Check sheet for the modelled part. Datum: model origin and axes. Units: mm. Face numbers are marked on the shaded views. Coordinates: 2 decimals unless noted, no trailing zeros. Loops run counter-clockwise (first coordinate to the right, second up) from the corner with the lowest first, then second, coordinate; pieces in that order, holes last. Notation, with made-up numbers: M -38,44 L -14,44 A30 ccw -14,75 Z; hole C 51.25,2.5 d2. An arc over 180 degrees is marked long. Use CSV: the item, a comma, the result in double quotes. Start each with the question number.
(1) Section check B-B on z = -15. Record the cut outline in (x, y), and give its area (3 significant figures).
(2) Section check A-A on x = 0. Record the cut outline in (y, z).
(3) Section check C-C on z = 0. Record the cut outline in (x, y).
(4) Go/stop test with flat-tipped pins: pin 1 Ø2.5 at (x, z) = (0, -15) entering from +Y (1 decimal); pin 2 Ø6.5 at (x, z) = (0, 15) entering from +Y; pin 3 Ø1 at (x, y) = (-3, 26) entering from +Z; pin 4 Ø10 at (y, z) = (21, 8) entering from -X. Record where each tip stops, or that it passes through.
(5) Section check D-D on y = -1. Record the cut outline in (x, z).
(6) Draft check along Z on the marked faces 1, 2 and 3. Enter one of: pulls with the +Z half, pulls with the -Z half, needs draft (parallel to the pull), parting line crosses it, or undercut.
(7) Scan lines: line 1 (Z direction, x = 0, y = -1.5); line 2 (X direction, y = 26, z = 0); line 3 (X direction, y = 0, z = 15). Record each from-to range of solid material in increasing order.
from build123d import *

# Parameters (mm, degrees)
SKETCH1_W           = 29
SKETCH1_H           = 7
BOSS_EXTRUDE1_DEPTH = 20
SKETCH2_R           = 2
CUT_EXTRUDE1_DEPTH  = 8
SKETCH3_R           = 7.75
SKETCH3_R_2         = 5.25
EXTRUDE_THIN1_DEPTH = 30


with BuildPart() as part:
    # Sketch1 → Boss-Extrude1 (new body, symmetric)
    with BuildSketch(Plane.XY):
        Rectangle(SKETCH1_W, SKETCH1_H)
    extrude(amount=BOSS_EXTRUDE1_DEPTH, both=True)

    # Sketch2 → Cut-Extrude1 (cut, through all)
    with BuildSketch(Plane(origin=(0, 3.5, 0), x_dir=(1, 0, 0), z_dir=(0, 1, 0))):
        with Locations((0, 15)):
            Circle(SKETCH2_R)
        with Locations((0, -15)):
            Circle(SKETCH2_R)
    extrude(amount=-CUT_EXTRUDE1_DEPTH, mode=Mode.SUBTRACT)

    # Sketch3 → Extrude-Thin1 (add)
    with BuildSketch(Plane(origin=(0, 3.5, 0), x_dir=(1, 0, 0), z_dir=(0, 1, 0))):
        Circle(SKETCH3_R)
        Circle(SKETCH3_R_2, mode=Mode.SUBTRACT)
    extrude(amount=EXTRUDE_THIN1_DEPTH)


solid = part.part
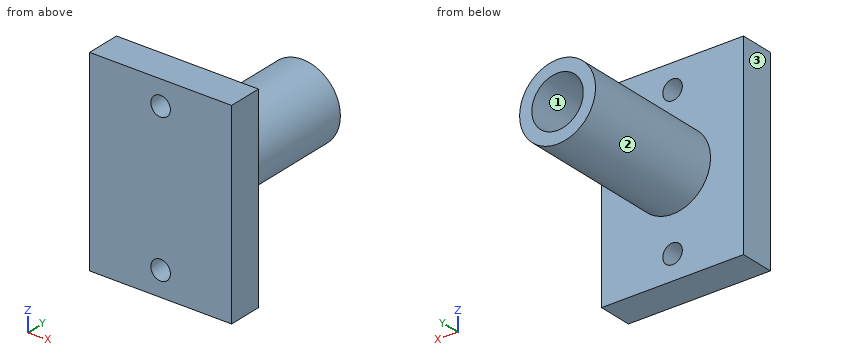
Outcome:
1,outline,"M -14.5,-3.5 L -2,-3.5 L -2,3.5 L -14.5,3.5 Z; M 2,-3.5 L 14.5,-3.5 L 14.5,3.5 L 2,3.5 Z"
1,area,"175 mm²"
2,outline,"M -3.5,-20 L 3.5,-20 L 3.5,-17 L -3.5,-17 Z; M -3.5,-13 L 3.5,-13 L 3.5,-7.75 L 33.5,-7.75 L 33.5,-5.25 L 3.5,-5.25 L 3.5,5.25 L 33.5,5.25 L 33.5,7.75 L 3.5,7.75 L 3.5,13 L -3.5,13 Z; M -3.5,17 L 3.5,17 L 3.5,20 L -3.5,20 Z"
3,outline,"M -14.5,-3.5 L 14.5,-3.5 L 14.5,3.5 L 7.75,3.5 L 7.75,33.5 L 5.25,33.5 L 5.25,3.5 L -5.25,3.5 L -5.25,33.5 L -7.75,33.5 L -7.75,3.5 L -14.5,3.5 Z"
4,pin 1,"passes through"
4,pin 2,"stops at y = 3.5"
4,pin 3,"stops at z = 7.34"
4,pin 4,"stops at x = -7.15"
5,outline,"M -14.5,-20 L 14.5,-20 L 14.5,20 L -14.5,20 Z; hole C 0,-15 d4; hole C 0,15 d4"
6,face 1,"undercut"
6,face 2,"parting line crosses it"
6,face 3,"needs draft"
7,line 1,"z = -20 to -17, -13 to 13, 17 to 20"
7,line 2,"x = -7.75 to -5.25, 5.25 to 7.75"
7,line 3,"x = -14.5 to -2, 2 to 14.5"
